Could you check a few things on this model? Use its own coordinates, in mm. Face numbers are marked on the shaded views. A direction names the side the tool comes from. Give positions to 0.01 mm unless a question says otherwise; leave off trailing zeros. Loops run counter-clockwise (first coordinate to the right, second up) from the corner with the lowest first, then second, coordinate; pieces in that order, holes last. Notation, with made-up numbers: M 28,80 L 67,80 A11 cw 67,94 Z; hole C 36.25,66.25 d9. An arc over 180 degrees is marked long. Use CSV: the item, a comma, the result in double quotes.
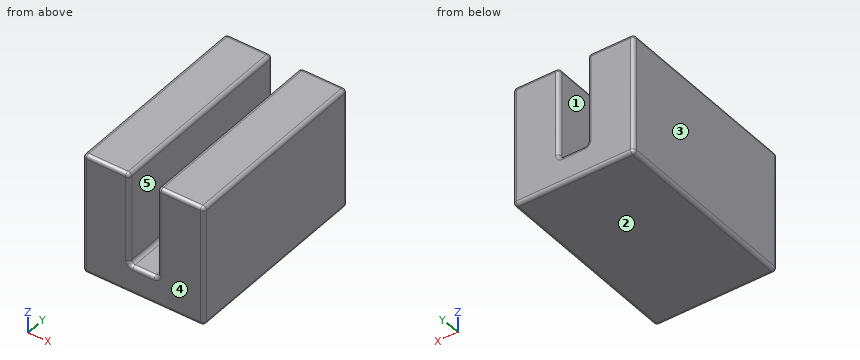
```python
from build123d import *

# Parameters (mm, degrees)
F0_W     = 33.147
F0_H     = 66.294
F1_DEPTH = 69.85
F2_R     = 2.54


with BuildPart() as f1:
    # F0 (on Front) → F1 (new body, symmetric)
    with BuildSketch(Plane.XZ):
        with Locations((-12.4733666049, 21.13100771)):
            Rectangle(F0_W, F0_H)
        Polygon((57.5671333951, -32.33599229), (57.5671333951, -12.01599229), (24.4201333951, -12.01599229), (4.1001333951, -12.01599229), (-29.0468666049, -12.01599229), (-29.0468666049, -32.33599229), align=None)
        with Locations((40.9936333951, 21.13100771)):
            Rectangle(F0_W, F0_H)
    extrude(amount=F1_DEPTH, both=True)

    # F2
    f2_edges = [f1.edges().sort_by_distance(p)[0] for p in [
        (-12.473367, 69.85, 54.278008),
        (-29.046867, 0, 54.278008),
        (-12.473367, -69.85, 54.278008),
        (4.100133, 0, 54.278008),
        (57.567133, 0, 54.278008),
        (40.993633, 69.85, 54.278008),
        (24.420133, 0, 54.278008),
        (40.993633, -69.85, 54.278008),
        (57.567133, 0, -32.335992),
        (57.567133, 69.85, 10.971008),
        (57.567133, -69.85, 10.971008),
        (24.420133, 0, -12.015992),
        (14.260133, 69.85, -12.015992),
        (4.100133, 0, -12.015992),
        (14.260133, -69.85, -12.015992),
        (4.100133, 69.85, 21.131008),
        (4.100133, -69.85, 21.131008),
        (-29.046867, 0, -32.335992),
        (14.260133, 69.85, -32.335992),
        (14.260133, -69.85, -32.335992),
        (-29.046867, 69.85, 10.971008),
        (-29.046867, -69.85, 10.971008),
        (24.420133, 69.85, 21.131008),
        (24.420133, -69.85, 21.131008),
    ]]
    fillet(f2_edges, radius=F2_R)


solid = f1.part
```
1. Which directions (+Z, -Z, +X, -X, +Y, -Y) give clear straight access to the entire face, cutting with the end or side of a thin tool? Please do the marked faces 4 and 5.
Outcome:
face 4,"+Z, -Z, +X, -X, -Y"
face 5,"+Z, +Y, -Y"
2. I want a section at B-B, the plane y = -61. List the corners of the cut face in (x, z) for me, then the cut area to 3 significant figures.
Outcome:
outline,"M -29.05,-29.8 A2.54 ccw -26.51,-32.34 L 55.03,-32.34 A2.54 ccw 57.57,-29.8 L 57.57,51.74 A2.54 ccw 55.03,54.28 L 26.96,54.28 A2.54 ccw 24.42,51.74 L 24.42,-9.48 A2.54 cw 21.88,-12.02 L 6.64,-12.02 A2.54 cw 4.1,-9.48 L 4.1,51.74 A2.54 ccw 1.56,54.28 L -26.51,54.28 A2.54 ccw -29.05,51.74 Z"
area,"6,150 mm2"
3. I want a section at A-A, the plane z = 27.5. List the corners of the cut face in (x, y) for me.
Outcome:
outline,"M -29.05,-67.31 A2.54 ccw -26.51,-69.85 L 1.56,-69.85 A2.54 ccw 4.1,-67.31 L 4.1,67.31 A2.54 ccw 1.56,69.85 L -26.51,69.85 A2.54 ccw -29.05,67.31 Z; M 24.42,-67.31 A2.54 ccw 26.96,-69.85 L 55.03,-69.85 A2.54 ccw 57.57,-67.31 L 57.57,67.31 A2.54 ccw 55.03,69.85 L 26.96,69.85 A2.54 ccw 24.42,67.31 Z"
4. Please list where these lines run through material, in increasing order: line 1 (X direction, y = 57, z = 6.5); line 2 (Z direction, x = 17, y = -5); line 3 (Z direction, x = 23.5, y = -51).
Outcome:
line 1,"-29.05 to 4.1, 24.42 to 57.57"
line 2,"-32.34 to -12.02"
line 3,"-32.34 to -11.43"
5. If we mould it in two halves opening along X, with no side actions, what happens to the marked faces 1, 2 and 3? For each: +X half, -X half, draft (parallel to the pull), parting line (faces both ways), or undercut.
Outcome:
face 1,"undercut"
face 2,"draft"
face 3,"-X half"
6. I'm going to push flat-ended pins straight in: pin 1 Ø3 at (x, y) = (22.5, -56) entering from +Z; pin 2 Ø12 at (x, y) = (11, -21.5) entering from +Z. Where does each tip first touch, or does it pass through?
Outcome:
pin 1,"z = -10.88"
pin 2,"z = -11.42"
